```python
from build123d import *

# Parameters (mm, degrees)
SKETCH1_R           = 2.5
BOSS_EXTRUDE1_DEPTH = 3.5
SKETCH2_R           = 1.25
BOSS_EXTRUDE2_DEPTH = 3


with BuildPart() as part:
    # Sketch1 → Boss-Extrude1 (new body)
    with BuildSketch(Plane(origin=(0, 0, 0), x_dir=(1, 0, 0), z_dir=(0, 1, 0))):
        with Locations(Location((0, 0, 0), (0, 0, 270))):
            Circle(SKETCH1_R)
    extrude(amount=BOSS_EXTRUDE1_DEPTH)

    # Sketch2 → Boss-Extrude2 (add)
    with BuildSketch(Plane(origin=(0, 3.5, 0), x_dir=(1, 0, 0), z_dir=(0, 1, 0))):
        with Locations(Location((0, 0, 0), (0, 0, 270))):
            Circle(SKETCH2_R)
    extrude(amount=BOSS_EXTRUDE2_DEPTH)

    # Sketch3 → Revolve1 (revolve)
    with BuildSketch(Plane.XY, mode=Mode.PRIVATE) as revolve1_sk:
        Polygon((1.25, 6.5), (1.25, 5.5), (1.45, 5.5), align=None)
    revolve(revolve1_sk.sketch.rotate(Axis((0, 0, 0), (0, 1, 0)), 90), axis=Axis((0, 0, 0), (0, 1, 0)))


solid = part.part
```
Read the model definition and answer for the solid it produces. Units are mm, in the model's axes. Coordinates: 2 decimals unless noted, no trailing zeros. Write each loop counter-clockwise with the first axis right and the second up, starting at its lowest first coordinate (ties: lowest second). Pieces come first, ordered by that corner, then holes. Notation, with made-up numbers: (1.25, 10) -> (44.25, 10) arc R20 cw to (44.25, 28) -> close; hole circle Ø8 at (-27, 17.25). An arc over 180 degrees is marked (long way). Return JSON: item names as keys, results as strings.
1. Each of these flat-tipped pins is pushed along its axis until it touches: P1, Ø1, axis at y = 0.5, z = 1.5, coming from the -X side; P2, Ø2, axis at x = 0, y = 5.5, coming from the -Z side; P3, Ø0.9, axis at x = -0.5, z = -0.5, coming from the -Y side. Where does it stop, or does it pass through?
Found:
{"P1": "x = -2.29", "P2": "z = -1.45", "P3": "y = 0"}
2. A cutting plane is placed at A-A (x = 0). Determine the outline of the cut face in (y, z), and give its area (3 significant figures).
Found:
{"outline": "(0, -2.5) -> (3.5, -2.5) -> (3.5, -1.25) -> (5.5, -1.25) -> (5.5, -1.45) -> (6.5, -1.25) -> (6.5, 1.25) -> (5.5, 1.45) -> (5.5, 1.25) -> (3.5, 1.25) -> (3.5, 2.5) -> (0, 2.5) -> close", "area": "25.2 mm2"}
3. Determine the mould class of faces 1 (the face through (0, 6.5, 0)), 2 (the face through (-1.22, 4.49, -0.27)), 3 (the face through (-2.44, 1.73, -0.54)), 4 (the face through (0, 0, 0)) for opening direction Y: pulls with the +Y half, pulls with the -Y half, needs draft (parallel to the pull), parting line crosses it, or undercut.
Found:
{"face 1": "pulls with the +Y half", "face 2": "undercut", "face 3": "needs draft", "face 4": "pulls with the -Y half"}
4. A cutting plane is placed at B-B (z = 0). Determine the outline of the cut face in (x, y), and give its area (3 significant figures).
Found:
{"outline": "(-2.5, 0) -> (2.5, 0) -> (2.5, 3.5) -> (1.25, 3.5) -> (1.25, 5.5) -> (1.45, 5.5) -> (1.25, 6.5) -> (-1.25, 6.5) -> (-1.45, 5.5) -> (-1.25, 5.5) -> (-1.25, 3.5) -> (-2.5, 3.5) -> close", "area": "25.2 mm2"}
5. Find the intervals of material crossed by line 1 along X through (y, z) = (1.5, 0.1); line 2 along Y through (x, z) = (-2.2, -0.35); line 3 along Z through (x, y) = (-0.7, 0.5), in increasing order. Write a range as from..to.
Found:
{"line 1": "-2.5..2.5", "line 2": "0..3.5", "line 3": "-2.4..2.4"}
6. A cutting plane is placed at C-C (y = 4). Determine the outline of the cut face in (x, z).
Found:
{"outline": "circle Ø2.5 at (0, 0)"}
7. A cutting plane is placed at D-D (y = 2.5). Determine the outline of the cut face in (x, z), and give its area (3 significant figures).
Found:
{"outline": "circle Ø5 at (0, 0)", "area": "19.6 mm2"}
